Here's the drawing with two shaded views (mm, measured from the low corner). I have some questions. A direction names the side the tool comes from. Give positions to 0.01 mm unless a question says otherwise; leave off trailing zeros. Write each loop counter-clockwise with the first axis right and the second up, starting at its lowest first coordinate (ties: lowest second). Pieces come first, ordered by that corner, then holes. Notation, with made-up numbers: (-38.75, -2.5) -> (10.25, -2.5) arc R25 ccw to (10.25, 10.5) -> close; hole circle Ø7 at (-7.75, 72.5). An arc over 180 degrees is marked (long way). One line per item, written item: value.
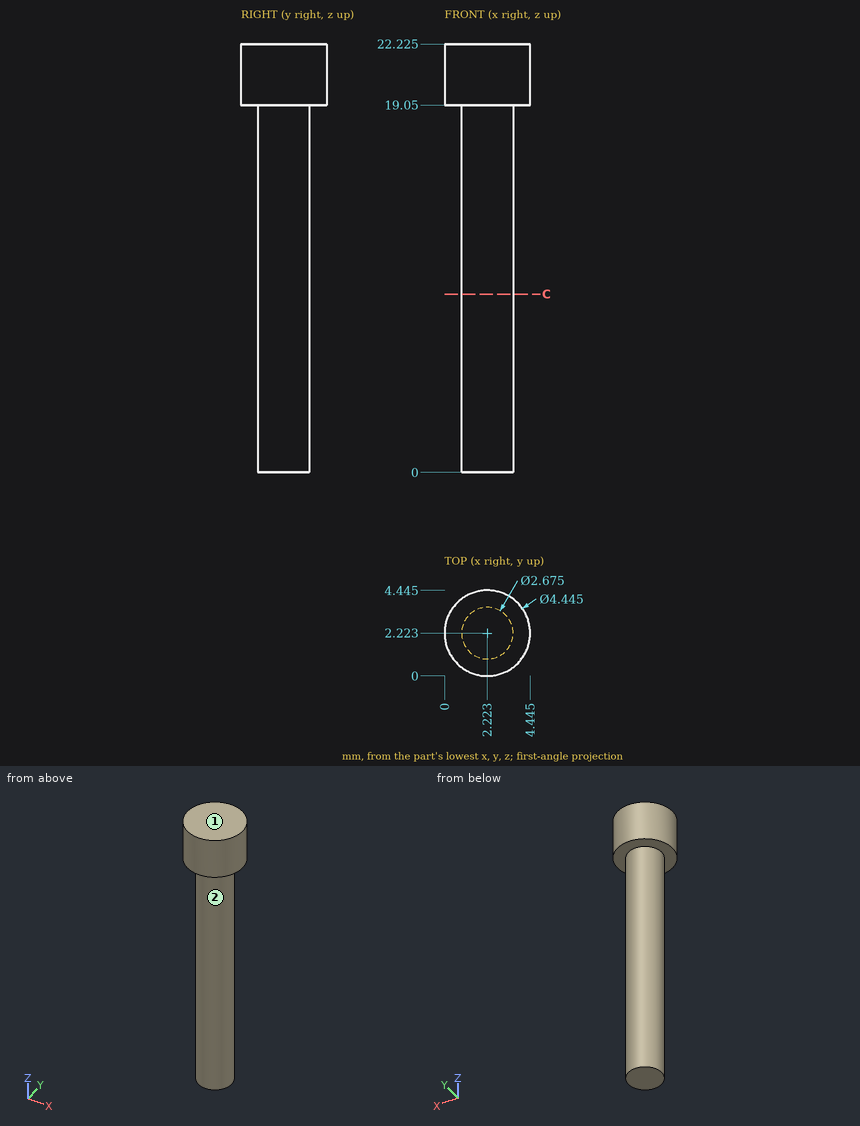
1) If we section it at C-C (z = 9.25): Write out the boundary of the cut face in (x, y) (1 decimal).
Answer list:
outline: circle Ø2.7 at (2.2, 2.2)
2) For the marked faces 1 and 2, which set-ups out of +Z, -Z, +X, -X, +Y, -Y let a thin tool reach every point of the face, with its end or its side?
Answer list:
face 1: +Z, +X, -X, +Y, -Y
face 2: -Z
3) Will this pin go through, and if not, where does the flat tip stop? pin 1 (2 mm diameter, centred on x = 2.5, z = 9.5, fed in from +Y).
Answer list:
pin 1: stops at y = 3.56
4) I need wall thicknesses on L1, parallel to Y at x = 3.25, z = 14.5 (1 decimal); L2, parallel to X at y = 1.15, z = 11.25 (1 decimal); L3, parallel to X at y = 2.15, z = 15. Which ranges of each line are inside material? Lowest first, please.
Answer list:
L1: y = 1.4 to 3.1
L2: x = 1.4 to 3
L3: x = 0.89 to 3.56
